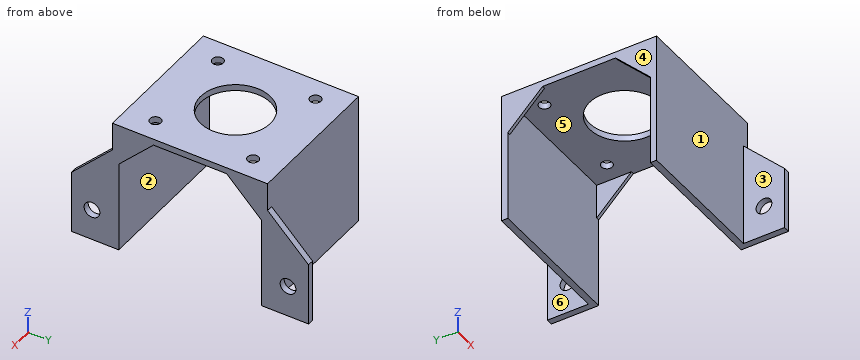
```python
from build123d import *

# Parameters (mm, degrees)
SKETCH1_W           = 45.2
SKETCH1_H           = 45.2
SKETCH1_R           = 1.75
SKETCH1_R_2         = 11.05
BOSS_EXTRUDE1_DEPTH = 2
SKETCH3_W           = 45.2
SKETCH3_H           = 2
BOSS_EXTRUDE2_DEPTH = 42
SKETCH4_W           = 20
SKETCH4_H           = 13
SKETCH4_R           = 2.5
BOSS_EXTRUDE3_DEPTH = 2
BOSS_EXTRUDE4_DEPTH = 1
BOSS_EXTRUDE5_DEPTH = 1


with BuildPart() as part:
    # Sketch1 → Boss-Extrude1 (new body)
    with BuildSketch(Plane.XY):
        Rectangle(SKETCH1_W, SKETCH1_H)
        with Locations((-15.5, 15.5)):
            Circle(SKETCH1_R, mode=Mode.SUBTRACT)
        with Locations((15.5, 15.5)):
            Circle(SKETCH1_R, mode=Mode.SUBTRACT)
        with Locations((-15.5, -15.5)):
            Circle(SKETCH1_R, mode=Mode.SUBTRACT)
        with Locations((15.5, -15.5)):
            Circle(SKETCH1_R, mode=Mode.SUBTRACT)
        Circle(SKETCH1_R_2, mode=Mode.SUBTRACT)
    extrude(amount=BOSS_EXTRUDE1_DEPTH)

    # Sketch3 → Boss-Extrude2 (add)
    with BuildSketch(Plane.XY.offset(2)):
        with Locations((0, 23.6)):
            Rectangle(SKETCH3_W, SKETCH3_H)
    boss_extrude2 = extrude(amount=-BOSS_EXTRUDE2_DEPTH)

    # Sketch4 → Boss-Extrude3 (add)
    with BuildSketch(Plane(origin=(22.6, 0, 0), x_dir=(0, 0, -1), z_dir=(1, 0, 0))):
        Polygon((7, 24.6), (20, 24.6), (20, 37.6), align=None)
        with Locations((30, 31.1)):
            Rectangle(SKETCH4_W, SKETCH4_H)
        with Locations((30, 31.1)):
            Circle(SKETCH4_R, mode=Mode.SUBTRACT)
    boss_extrude3 = extrude(amount=-BOSS_EXTRUDE3_DEPTH)

    # Mirror1: Boss-Extrude2, Boss-Extrude3 across plane
    add(boss_extrude2.mirror(Plane.ZX))
    add(boss_extrude3.mirror(Plane.ZX))

    # Sketch5 → Boss-Extrude4 (add)
    with BuildSketch(Plane.ZY.offset(22.6)):
        Polygon((-13, 24.6), (2, 9.6), (2, 24.6), align=None)
        Polygon((-13, -24.6), (2, -9.6), (2, -24.6), align=None)
    extrude(amount=-BOSS_EXTRUDE4_DEPTH)

    # Sketch6 → Boss-Extrude5 (add)
    with BuildSketch(Plane(origin=(22.6, 0, 0), x_dir=(0, 0, -1), z_dir=(1, 0, 0))):
        Polygon((-2, 9.6), (13, 24.6), (-2, 24.6), align=None)
        Polygon((13, -24.6), (-2, -9.6), (-2, -24.6), align=None)
    extrude(amount=-BOSS_EXTRUDE5_DEPTH)


solid = part.part
```
Input: part model. Units: mm. Frame: model coordinates. Face numbers are marked on the shaded views. A direction names the side the tool comes from. Coordinates: 2 decimals unless noted, no trailing zeros. Order: outer loops, then holes, each group sorted by start corner. A loop starts at its lowest first (then second) coordinate and runs counter-clockwise, first axis right, second up. Notation, with made-up numbers: (26.25, -14.5) - (53.25, -14.5) arc R17 cw to (53.25, -5.5) - close; hole circle Ø10 at (-32, 3.25). An arc over 180 degrees is marked (long way). Return JSON: item names as keys, results as strings.
Q1. Cut plane B-B (x = -15.5). Return loops of the section in (y, z).
The answers:
{"outline": "(-24.6, -40) - (-22.6, -40) - (-22.6, 0) - (-17.25, 0) - (-17.25, 2) - (-24.6, 2) - close; (-13.75, 0) - (13.75, 0) - (13.75, 2) - (-13.75, 2) - close; (17.25, 0) - (22.6, 0) - (22.6, -40) - (24.6, -40) - (24.6, 2) - (17.25, 2) - close"}
Q2. Draft query along X for the marked faces 1, 2 and 3. Return one class per face: +X half, -X half, draft (parallel to the pull), parting line (faces both ways), or undercut.
The answers:
{"face 1": "draft", "face 2": "undercut", "face 3": "-X half"}
Q3. First-contact query: pin 1 (12.5 mm diameter, centred on x = 8.5, z = -24, fed in from +Y); pin 2 (12 mm diameter, centred on x = -0.5, z = -30.5, fed in from -Y); pin 3 (4 mm diameter, centred on x = -11.5, y = 14, fed in from -Z); pin 4 (6 mm diameter, centred on y = -31.1, z = -30, fed in from +X). Flat tips, straight axial feed; report the tip coordinate or a pass-through.
The answers:
{"pin 1": "stops at y = 24.6", "pin 2": "stops at y = -24.6", "pin 3": "stops at z = 0", "pin 4": "stops at x = 22.6"}
Q4. Ray query, probe 1 along X at (y, z) = (15, 1); probe 2 along X at (y, z) = (19, -6); probe 3 along Y at (x, z) = (-15, 1). Return the intervals inside material, ascending.
The answers:
{"probe 1": "x = -22.6 to -17.18, -13.82 to 13.82, 17.18 to 22.6", "probe 2": "x = -22.6 to -21.6, 21.6 to 22.6", "probe 3": "y = -24.6 to -17.18, -13.82 to 13.82, 17.18 to 24.6"}
Q5. Cut plane A-A (z = -31.5). Return loops of the section in (x, y), then the cut area to 3 significant figures.
The answers:
{"outline": "(-22.6, -24.6) - (20.6, -24.6) - (20.6, -29.1) - (22.6, -29.1) - (22.6, -22.6) - (-22.6, -22.6) - close; (-22.6, 22.6) - (22.6, 22.6) - (22.6, 29.1) - (20.6, 29.1) - (20.6, 24.6) - (-22.6, 24.6) - close; (20.6, -37.6) - (22.6, -37.6) - (22.6, -33.1) - (20.6, -33.1) - close; (20.6, 33.1) - (22.6, 33.1) - (22.6, 37.6) - (20.6, 37.6) - close", "area": "217 mm2"}
Q6. Access query for the marked faces 4, 5 and 6. Directions: +Z, -Z, +X, -X, +Y, -Y. A direction counts if a zero-diameter tool reaches every point of the face in a straight line with its end or side. Return the directions, or none.
The answers:
{"face 4": "+Z, -Z, -X, +Y, -Y", "face 5": "-Z", "face 6": "+Z, -Z, -X, +Y"}
Q7. Cut plane C-C (x = 7). Return loops of the section in (y, z).
The answers:
{"outline": "(-24.6, -40) - (-22.6, -40) - (-22.6, 0) - (-8.55, 0) - (-8.55, 2) - (-24.6, 2) - close; (8.55, 0) - (22.6, 0) - (22.6, -40) - (24.6, -40) - (24.6, 2) - (8.55, 2) - close"}
Q8. Cut plane D-D (y = -5). Return loops of the section in (x, z).
The answers:
{"outline": "(-22.6, 0) - (-9.85, 0) - (-9.85, 2) - (-22.6, 2) - close; (9.85, 0) - (22.6, 0) - (22.6, 2) - (9.85, 2) - close"}
